Part model, mm, in its own coordinate system. A direction names the side the tool comes from. Coordinates: 2 decimals unless noted, no trailing zeros. Loops run counter-clockwise (first coordinate to the right, second up) from the corner with the lowest first, then second, coordinate; pieces in that order, holes last. Notation, with made-up numbers: (17, 28) -> (66, 28) arc R30 cw to (66, 60) -> close; hole circle Ø3 at (84.5, -15.75). An arc over 180 degrees is marked (long way). One line per item, written item: value. Start each with the question number.
from build123d import *

# Parameters (mm, degrees)
SKETCH1_R               = 20
SKETCH1_R_2             = 6
SKETCH1_R_3             = 1.5
BOSS_EXTRUDE1_DEPTH     = 5
SKETCH2_R               = 9
SKETCH2_R_2             = 6
BOSS_EXTRUDE2_DEPTH     = 10
SKETCH3_R               = 50
BOSS_EXTRUDE3_DEPTH     = 2
CUT_EXTRUDE1_START      = -2
CUT_EXTRUDE1_DEPTH      = 2
CUT_EXTRUDE2_DEPTH      = 72.944422994
CUT_EXTRUDE2_DEPTH_BACK = 72.944422994
SKETCH5_R               = 1.5


with BuildPart() as part:
    # Sketch1 → Boss-Extrude1 (new body)
    with BuildSketch(Plane.XY):
        Circle(SKETCH1_R)
        Circle(SKETCH1_R_2, mode=Mode.SUBTRACT)
        with Locations((-10.061951403, 10.061951403)):
            Circle(SKETCH1_R_3, mode=Mode.SUBTRACT)
        with Locations(Location((10.061951403, 10.061951403, 0), (0, 0, 180))):
            Circle(SKETCH1_R_3, mode=Mode.SUBTRACT)
        with Locations((10.061951403, -10.061951403)):
            Circle(SKETCH1_R_3, mode=Mode.SUBTRACT)
        with Locations(Location((-10.061951403, -10.061951403, 0), (0, 0, 180))):
            Circle(SKETCH1_R_3, mode=Mode.SUBTRACT)
    extrude(amount=BOSS_EXTRUDE1_DEPTH)

    # Sketch2 → Boss-Extrude2 (add)
    with BuildSketch(Plane.XY.offset(5)):
        Circle(SKETCH2_R)
        Circle(SKETCH2_R_2, mode=Mode.SUBTRACT)
    extrude(amount=BOSS_EXTRUDE2_DEPTH)

    # Sketch3 → Boss-Extrude3 (add)
    with BuildSketch(Plane.XY.offset(5)):
        Circle(SKETCH3_R)
    extrude(amount=BOSS_EXTRUDE3_DEPTH)

    # Sketch4 → Cut-Extrude1 (cut)
    with BuildSketch(Plane.XY.offset(7).offset(CUT_EXTRUDE1_START)):
        with BuildLine():
            Line((-7, 49.507575178), (-7, 34.507575178))
            ThreePointArc((-7, 34.507575178), (0, 27.507575178), (7, 34.507575178))
            Line((7, 34.507575178), (7, 49.507575178))
            ThreePointArc((7, 49.507575178), (0, 50), (-7, 49.507575178))
        make_face()
        with BuildLine():
            Line((39.374817784, 30.815965415), (26.384436727, 23.315965415))
            ThreePointArc((26.384436727, 23.315965415), (23.822258901, 13.753787589), (33.384436727, 11.191609762))
            Line((33.384436727, 11.191609762), (46.374817784, 18.691609762))
            ThreePointArc((46.374817784, 18.691609762), (43.301270189, 25), (39.374817784, 30.815965415))
        make_face()
        with BuildLine():
            Line((46.374817784, -18.691609762), (33.384436727, -11.191609762))
            ThreePointArc((33.384436727, -11.191609762), (23.822258901, -13.753787589), (26.384436727, -23.315965415))
            Line((26.384436727, -23.315965415), (39.374817784, -30.815965415))
            ThreePointArc((39.374817784, -30.815965415), (43.301270189, -25), (46.374817784, -18.691609762))
        make_face()
        with BuildLine():
            Line((7, -49.507575178), (7, -34.507575178))
            ThreePointArc((7, -34.507575178), (0, -27.507575178), (-7, -34.507575178))
            Line((-7, -34.507575178), (-7, -49.507575178))
            ThreePointArc((-7, -49.507575178), (0, -50), (7, -49.507575178))
        make_face()
        with BuildLine():
            Line((-39.374817784, -30.815965415), (-26.384436727, -23.315965415))
            ThreePointArc((-26.384436727, -23.315965415), (-23.822258901, -13.753787589), (-33.384436727, -11.191609762))
            Line((-33.384436727, -11.191609762), (-46.374817784, -18.691609762))
            ThreePointArc((-46.374817784, -18.691609762), (-43.301270189, -25), (-39.374817784, -30.815965415))
        make_face()
        with BuildLine():
            Line((-46.374817784, 18.691609762), (-33.384436727, 11.191609762))
            ThreePointArc((-33.384436727, 11.191609762), (-23.822258901, 13.753787589), (-26.384436727, 23.315965415))
            Line((-26.384436727, 23.315965415), (-39.374817784, 30.815965415))
            ThreePointArc((-39.374817784, 30.815965415), (-43.301270189, 25), (-46.374817784, 18.691609762))
        make_face()
    extrude(amount=CUT_EXTRUDE1_DEPTH, mode=Mode.SUBTRACT)

    # Sketch5 → Cut-Extrude2 (cut, two sides: drawn at the far end of the back side and taken through both)
    with BuildSketch(Plane(origin=(0, 0, 0), x_dir=(-1, 0, 0), z_dir=(0, 0, -1)).offset(-CUT_EXTRUDE2_DEPTH_BACK)):
        with Locations((-10.061951403, 10.061951403)):
            Circle(SKETCH5_R)
        with Locations(Location((-10.061951403, -10.061951403, 0), (0, 0, 180))):
            Circle(SKETCH5_R)
        with Locations(Location((10.061951403, 10.061951403, 0), (0, 0, 180))):
            Circle(SKETCH5_R)
        with Locations((10.061951403, -10.061951403)):
            Circle(SKETCH5_R)
    extrude(amount=CUT_EXTRUDE2_DEPTH + CUT_EXTRUDE2_DEPTH_BACK, mode=Mode.SUBTRACT)


solid = part.part
1) Slice it at C-C (z = 8.5). Give the cut face in (x, y).
2) Slice it at D-D (y = -15). Give the cut face in (x, z), then the cut area to 3 significant figures.
3) Slice it at A-A (y = 0). Give the cut face in (x, z), then the cut area to 3 significant figures.
4) Pin check, flat tips, straight feed: pin 1 Ø1 at (y, z) = (-44.5, 6.5) entering from +X; pin 2 Ø5 at (y, z) = (32, 6.5) entering from -X; pin 3 Ø1 at (y, z) = (43, 5.5) entering from +X; pin 4 Ø2 at (x, y) = (39.5, -28) entering from +Z. Stop position of each tip, or through.
5) Slice it at B-B (x = 0). Give the cut face in (y, z), then the cut area to 3 significant figures.
6) Pull direction X, two halves, no side cores. Call faces 1 (the cylindrical face through (-23.747, -13.888, 5.986)), 2 (the flat face through (-32.789, 27.013, 5.986)), 3 (the cylindrical face through (-0.15, 27.51, 5.99)), 4 (the cylindrical face through (24.767, -43.435, 5.986)): +X half, -X half, draft (parallel to the pull), parting line (faces both ways), or undercut.
7) Probe line 1 (Y direction, x = 0, z = 1.85); line 2 (Y direction, x = 0, z = 10.5). List the from-to ranges inside material, lowest first. Write a range as from..to.
8) Tool access for faces 5 (the cylindrical face through (-50, 0, 6)), 6 (the flat face through (32.789, -27.013, 5.986)), 7 (the flat face through (-39.79, -14.89, 5.99)), 8 (the cylindrical face through (-25.232, -43.167, 5.986)), 9 (the cylindrical face through (-4.336, -19.524, 2.465)): list every direction of +Z, -Z, +X, -X, +Y, -Y with a clear straight run to the whole face (end or side of a thin tool).
Check sheet entries:
1. outline: circle Ø18 at (0, 0); hole circle Ø12 at (0, 0)
2. outline: (-47.7, 5) -> (-39.98, 5) -> (-39.98, 7) -> (-47.7, 7) -> close; (-23.26, 5) -> (-13.23, 5) -> (-13.23, 0) -> (13.23, 0) -> (13.23, 5) -> (23.26, 5) -> (23.26, 7) -> (-23.26, 7) -> close; (39.98, 5) -> (47.7, 5) -> (47.7, 7) -> (39.98, 7) -> close
2. area: 256 mm^2
3. outline: (-50, 5) -> (-20, 5) -> (-20, 0) -> (-6, 0) -> (-6, 5) -> (6, 5) -> (6, 0) -> (20, 0) -> (20, 5) -> (50, 5) -> (50, 7) -> (9, 7) -> (9, 15) -> (6, 15) -> (6, 7) -> (-6, 7) -> (-6, 15) -> (-9, 15) -> (-9, 7) -> (-50, 7) -> close
3. area: 388 mm^2
4. pin 1: stops at x = 23.75
4. pin 2: stops at x = -39.37
4. pin 3: stops at x = 26.34
4. pin 4: passes through
5. outline: (-27.51, 5) -> (-20, 5) -> (-20, 0) -> (-6, 0) -> (-6, 5) -> (6, 5) -> (6, 0) -> (20, 0) -> (20, 5) -> (27.51, 5) -> (27.51, 7) -> (9, 7) -> (9, 15) -> (6, 15) -> (6, 7) -> (-6, 7) -> (-6, 15) -> (-9, 15) -> (-9, 7) -> (-27.51, 7) -> close
5. area: 298 mm^2
6. face 1: undercut
6. face 2: -X half
6. face 3: undercut
6. face 4: +X half
7. line 1: y = -20..-6, 6..20
7. line 2: y = -9..-6, 6..9
8. face 5: +Z, -Z, -X
8. face 6: +Z, -Z, +X
8. face 7: +Z, -Z
8. face 8: +Z, -Z, -X, -Y
8. face 9: -Z
